```python
from build123d import *

# Parameters (mm, degrees)
F0_W           = 67.1
F0_H           = 38.6
F1_DEPTH       = 7
F2_DEPTH       = 5
F3_D           = 2.2
F3_CSINK_D     = 6.72
F3_CSINK_ANGLE = 90
F5_D           = 2.2


with BuildPart() as f1:
    # F0 (on Top) → F1 (new body)
    with BuildSketch(Plane.XY):
        with BuildLine():
            ThreePointArc((40.55, 16.8), (39.231981, 19.981981), (36.05, 21.3))
            Line((36.05, 21.3), (-36.05, 21.3))
            ThreePointArc((-36.05, 21.3), (-39.231981, 19.981981), (-40.55, 16.8))
            Line((-40.55, 16.8), (-40.55, -16.8))
            ThreePointArc((-40.55, -16.8), (-39.231981, -19.981981), (-36.05, -21.3))
            Line((-36.05, -21.3), (36.05, -21.3))
            ThreePointArc((36.05, -21.3), (39.231981, -19.981981), (40.55, -16.8))
            Line((40.55, -16.8), (40.55, 16.8))
        make_face()
        Rectangle(F0_W, F0_H, mode=Mode.SUBTRACT)
    extrude(amount=F1_DEPTH)

    # F0 (on Top) → F2 (join)
    with BuildSketch(Plane.XY):
        with BuildLine():
            Line((42.55, -16.8), (42.55, 16.8))
            ThreePointArc((42.55, 16.8), (40.646194, 21.396194), (36.05, 23.3))
            Line((36.05, 23.3), (-36.05, 23.3))
            ThreePointArc((-36.05, 23.3), (-40.646194, 21.396194), (-42.55, 16.8))
            Line((-42.55, 16.8), (-42.55, -16.8))
            ThreePointArc((-42.55, -16.8), (-40.646194, -21.396194), (-36.05, -23.3))
            Line((-36.05, -23.3), (36.05, -23.3))
            ThreePointArc((36.05, -23.3), (40.646194, -21.396194), (42.55, -16.8))
        make_face()
        with BuildLine():
            Line((-36.05, 21.3), (36.05, 21.3))
            ThreePointArc((36.05, 21.3), (39.231981, 19.981981), (40.55, 16.8))
            Line((40.55, 16.8), (40.55, -16.8))
            ThreePointArc((40.55, -16.8), (39.231981, -19.981981), (36.05, -21.3))
            Line((36.05, -21.3), (-36.05, -21.3))
            ThreePointArc((-36.05, -21.3), (-39.231981, -19.981981), (-40.55, -16.8))
            Line((-40.55, -16.8), (-40.55, 16.8))
            ThreePointArc((-40.55, 16.8), (-39.231981, 19.981981), (-36.05, 21.3))
        make_face(mode=Mode.SUBTRACT)
    extrude(amount=F2_DEPTH)

    # F3 (through all)
    with Locations(Plane(origin=(0, 0, 0), x_dir=(1, 0, 0), z_dir=(0, 0, -1))):
        with Locations((37.2, 14.05), (37.2, -14.05), (-37.2, -14.05), (-37.2, 14.05)):
            CounterSinkHole(F3_D / 2, F3_CSINK_D / 2, counter_sink_angle=F3_CSINK_ANGLE)

    # F5 (through all)
    with Locations(Plane.YZ.offset(42.55)):
        with Locations((0, 2.5)):
            Hole(F5_D / 2)


solid = f1.part
```
Model file for the job. Use its own axes, mm. A direction names the side the tool comes from. Give positions to 0.01 mm unless a question says otherwise; leave off trailing zeros. Loops run counter-clockwise (first coordinate to the right, second up) from the corner with the lowest first, then second, coordinate; pieces in that order, holes last. Notation, with made-up numbers: (23.5, 15) - (36.5, 15) arc R25 ccw to (36.5, 45) - close; hole circle Ø1 at (83, -16.75). An arc over 180 degrees is marked (long way). One line per item, written item: value. Start each with the question number.
1. Which spindle directions (+Z, -Z, +X, -X, +Y, -Y) get a long thin tool onto all of the face, cutting with end or side? Do faces 4 (the flat face through (0, -22, 5)), 5 (the flat face through (33.55, 0, 4)), 6 (the cylindrical face through (39.267, 19.947, 5.986)). Say none if no direction does.
2. Slice it at A-A (x = -5). List the corners of the cut face in (y, z), plus the area to 3 significant figures.
3. Probe L1, parallel to Y at x = -15.5, z = 3.75; L2, parallel to X at y = -14.05, z = 3.7; L3, parallel to Z at x = -39, y = 0. List the from-to ranges inside material, lowest first. Write a range as from..to.
4. Slice it at C-C (y = 9). List the corners of the cut face in (x, z).
5. Pin check, flat tips, straight feed: pin 1 (2 mm diameter, centred on x = 37.2, y = -14.05, fed in from +Z); pin 2 (1.6 mm diameter, centred on x = 9.5, z = 6, fed in from +Y); pin 3 (0.6 mm diameter, centred on x = 5.5, z = 6.5, fed in from -Y); pin 4 (0.6 mm diameter, centred on y = 4.5, z = 5.5, fed in from +X). Stop position of each tip, or through.
6. Slice it at B-B (y = 14.05). List the corners of the cut face in (x, z).
7. Pull direction Y, two halves, no side cores. Call faces 1 (the cylindrical face through (40.696, 21.345, 2.465)), 2 (the cylindrical face through (-40.696, -21.345, 2.465)), 3 (the cylindrical face through (37.99, -0.59, 3.43)): pulls with the +Y half, pulls with the -Y half, needs draft (parallel to the pull), parting line crosses it, or undercut.
8. Slice it at D-D (x = 37.2). List the corners of the cut face in (y, z).
Solution:
1. face 4: +Z
1. face 5: +Z, -Z
1. face 6: +Z, +X, +Y
2. outline: (-23.3, 0) - (-19.3, 0) - (-19.3, 7) - (-21.3, 7) - (-21.3, 5) - (-23.3, 5) - close; (19.3, 0) - (23.3, 0) - (23.3, 5) - (21.3, 5) - (21.3, 7) - (19.3, 7) - close
2. area: 48.0 mm^2
3. L1: y = -23.3..-19.3, 19.3..23.3
3. L2: x = -42.55..-38.3, -36.1..-33.55, 33.55..36.1, 38.3..42.55
3. L3: z = 0..1.4, 3.6..7
4. outline: (-42.55, 0) - (-33.55, 0) - (-33.55, 7) - (-40.55, 7) - (-40.55, 5) - (-42.55, 5) - close; (33.55, 0) - (42.55, 0) - (42.55, 5) - (40.55, 5) - (40.55, 7) - (33.55, 7) - close
5. pin 1: passes through
5. pin 2: stops at y = 21.3
5. pin 3: stops at y = -21.3
5. pin 4: stops at x = 40.55
6. outline: (-42.55, 0) - (-40.56, 0) - (-38.3, 2.26) - (-38.3, 7) - (-40.55, 7) - (-40.55, 5) - (-42.55, 5) - close; (-36.1, 2.26) - (-33.84, 0) - (-33.55, 0) - (-33.55, 7) - (-36.1, 7) - close; (33.55, 0) - (33.84, 0) - (36.1, 2.26) - (36.1, 7) - (33.55, 7) - close; (38.3, 2.26) - (40.56, 0) - (42.55, 0) - (42.55, 5) - (40.55, 5) - (40.55, 7) - (38.3, 7) - close
7. face 1: pulls with the +Y half
7. face 2: pulls with the -Y half
7. face 3: undercut
8. outline: (-23.2, 0) - (-17.41, 0) - (-15.15, 2.26) - (-15.15, 7) - (-21.15, 7) - (-21.15, 5) - (-23.2, 5) - close; (-12.95, 2.26) - (-10.69, 0) - (10.69, 0) - (12.95, 2.26) - (12.95, 7) - (-12.95, 7) - close; (15.15, 2.26) - (17.41, 0) - (23.2, 0) - (23.2, 5) - (21.15, 5) - (21.15, 7) - (15.15, 7) - close; hole circle Ø2.2 at (0, 2.5)
